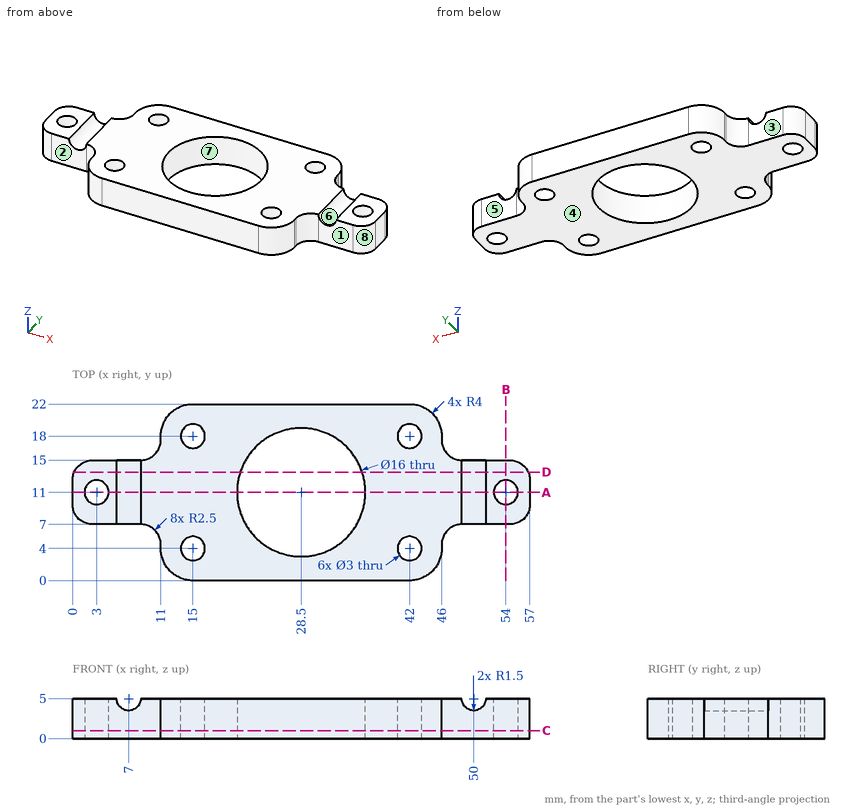
Input: dimensioned drawing with shaded views. Units: mm. Origin: part minimum x, y, z. A direction names the side the tool comes from. Coordinates: 2 decimals unless noted, no trailing zeros. Order: outer loops, then holes, each group sorted by start corner. A loop starts at its lowest first (then second) coordinate and runs counter-clockwise, first axis right, second up.
(1) Access query for the marked faces 1, 2, 3, 4 and 5. Directions: +Z, -Z, +X, -X, +Y, -Y. A direction counts if a zero-diameter tool reaches every point of the face in a straight line with its end or side. Return the directions, or none.
(2) Section query D-D (y = 13.5). Return the cut outline in (x, z).
(3) Material intervals for probe 1 along Y at (x, z) = (15, 2.15); probe 2 along Y at (x, z) = (3, 4); probe 3 along X at (y, z) = (8.25, 4.3), sorted ascending.
(4) Section query A-A (y = 11). Return the cut outline in (x, z), plus the area to 3 significant figures.
(5) Section query C-C (z = 1). State how many separate pieces and enclosed holes the cut face has, plus the area to 3 significant figures.
(6) First-contact query: pin 1 (2 mm diameter, centred on x = 46.5, z = 3.5, fed in from -Y); pin 2 (0.6 mm diameter, centred on y = 18, z = 3.5, fed in from +X). Flat tips, straight axial feed; report the tip coordinate or a pass-through.
(7) Section query B-B (x = 54). Return the cut outline in (y, z), plus the area to 3 significant figures.
(8) Draft query along Y for the marked faces 6, 7 and 8. Return one class per face: pulls with the +Y half, pulls with the -Y half, needs draft (parallel to the pull), parting line crosses it, or undercut.
Solution:
1. face 1: +Z, -Z, +X, -Y
1. face 2: +Z, -Z, -X, -Y
1. face 3: +Z, -Z, -X, +Y
1. face 4: -Z, +X, -X, +Y, -Y
1. face 5: +Z, -Z, +X, +Y
2. outline: (0.21, 0) - (20.9, 0) - (20.9, 5) - (8.5, 5) arc R1.5 cw to (5.5, 5) - (0.21, 5) - close; (36.1, 0) - (56.79, 0) - (56.79, 5) - (51.5, 5) arc R1.5 cw to (48.5, 5) - (36.1, 5) - close
3. probe 1: y = 0 to 2.5, 5.5 to 16.5, 19.5 to 22
3. probe 2: y = 7 to 9.5, 12.5 to 15
3. probe 3: x = 0.33 to 5.67, 8.33 to 20.99, 36.01 to 48.67, 51.33 to 56.67
4. outline: (0, 0) - (1.5, 0) - (1.5, 5) - (0, 5) - close; (4.5, 0) - (20.5, 0) - (20.5, 5) - (8.5, 5) arc R1.5 cw to (5.5, 5) - (4.5, 5) - close; (36.5, 0) - (52.5, 0) - (52.5, 5) - (51.5, 5) arc R1.5 cw to (48.5, 5) - (36.5, 5) - close; (55.5, 0) - (57, 0) - (57, 5) - (55.5, 5) - close
4. area: 168 mm2
5. separate pieces: 1
5. enclosed holes: 7
5. area: 689 mm2
6. pin 1: stops at y = 2.06
6. pin 2: stops at x = 46
7. outline: (7, 0) - (9.5, 0) - (9.5, 5) - (7, 5) - close; (12.5, 0) - (15, 0) - (15, 5) - (12.5, 5) - close
7. area: 25.0 mm2
8. face 6: needs draft
8. face 7: undercut
8. face 8: pulls with the -Y half
